from build123d import *

# Parameters (mm, degrees)
SKETCH_1_R          = 18.5
EXTRUDE_1_DEPTH     = 24
SKETCH_2_R          = 6
EXTRUDE_2_DEPTH     = 6
SKETCH_3_R          = 3
EXTRUDE_3_DEPTH     = 15.5
SKETCH_4_R          = 17.5
EXTRUDE_4_DEPTH     = 30
SKETCH_5_R          = 10
EXTRUDE_6_DEPTH     = 11.5
CUT_EXTRUDE_1_DEPTH = 12
SKETCH_7_R          = 1.5
CUT_EXTRUDE_2_DEPTH = 10


with BuildPart() as part:
    # 草图1 → 凸台-拉伸1 (new body)
    with BuildSketch(Plane(origin=(0, 0, 0), x_dir=(1, 0, 0), z_dir=(0, 1, 0))):
        with Locations(Location((0, 0, 0), (0, 0, 270))):
            Circle(SKETCH_1_R)
    extrude(amount=EXTRUDE_1_DEPTH)

    # 草图2 → 凸台-拉伸2 (add)
    with BuildSketch(Plane(origin=(0, 24, 0), x_dir=(1, 0, 0), z_dir=(0, 1, 0))):
        with Locations(Location((0, 7, 0), (0, 0, 270))):
            Circle(SKETCH_2_R)
    extrude(amount=EXTRUDE_2_DEPTH)

    # 草图3 → 凸台-拉伸3 (add)
    with BuildSketch(Plane(origin=(0, 30, 0), x_dir=(1, 0, 0), z_dir=(0, 1, 0))):
        with Locations(Location((0, 7, 0), (0, 0, 270))):
            Circle(SKETCH_3_R)
    extrude(amount=EXTRUDE_3_DEPTH)

    # 草图4 → 凸台-拉伸4 (add)
    with BuildSketch(Plane.XZ):
        with Locations(Location((0, 0, 0), (0, 0, 90))):
            Circle(SKETCH_4_R)
    extrude(amount=EXTRUDE_4_DEPTH)

    # 草图5 → 凸台-拉伸6 (add)
    with BuildSketch(Plane.XZ.offset(30)):
        with Locations(Location((0, 0, 0), (0, 0, 270))):
            Circle(SKETCH_5_R)
    extrude(amount=EXTRUDE_6_DEPTH)

    # 草图6 → 切除-拉伸1 (cut)
    with BuildSketch(Plane(origin=(0, 45.5, 0), x_dir=(1, 0, 0), z_dir=(0, 1, 0))):
        with BuildLine():
            Line((-3.711279789, 9.5), (4.099560016, 9.5))
            ThreePointArc((4.099560016, 9.5), (0.194140114, 13.405419903), (-3.711279789, 9.5))
        make_face()
    extrude(amount=-CUT_EXTRUDE_1_DEPTH, mode=Mode.SUBTRACT)

    # 草图7 → 切除-拉伸2 (cut)
    with BuildSketch(Plane(origin=(0, 24, 0), x_dir=(1, 0, 0), z_dir=(0, 1, 0))):
        with Locations(Location((-15.5, 0, 0), (0, 0, 270))):
            Circle(SKETCH_7_R)
        with Locations(Location((-7.75, 13.423393759, 0), (0, 0, 270))):
            Circle(SKETCH_7_R)
        with Locations(Location((7.75, 13.423393759, 0), (0, 0, 270))):
            Circle(SKETCH_7_R)
        with Locations(Location((15.5, 0, 0), (0, 0, 270))):
            Circle(SKETCH_7_R)
        with Locations(Location((7.75, -13.423393759, 0), (0, 0, 270))):
            Circle(SKETCH_7_R)
        with Locations(Location((-7.75, -13.423393759, 0), (0, 0, 270))):
            Circle(SKETCH_7_R)
    extrude(amount=-CUT_EXTRUDE_2_DEPTH, mode=Mode.SUBTRACT)


solid = part.part
Model file for the job. Use its own axes, mm. A direction names the side the tool comes from. Give positions to 0.01 mm unless a question says otherwise; leave off trailing zeros. Order: outer loops, then holes, each group sorted by start corner. A loop starts at its lowest first (then second) coordinate and runs counter-clockwise, first axis right, second up. Notation, with made-up numbers: M 43.5,21.25 L 59.5,21.25 A16 ccw 59.5,42.25 Z; hole C 1,75 d10. An arc over 180 degrees is marked long. Write item = value, one per line.
Q1. Flat gauge pins, fed straight in: pin 1 (6 mm diameter, centred on x = 12, z = 5.5, fed in from +Y); pin 2 (1.5 mm diameter, centred on x = 8, z = 13, fed in from +Y); pin 3 (1.7 mm diameter, centred on x = 0.5, y = 40.5, fed in from -Z). Where does each tip first touch, or does it go through?
Derived:
pin_1 = 24
pin_2 = 14
pin_3 = -9.5
Q2. Cut at D-D, the plane z = -5. List the corners of the cut face in (x, y).
Derived:
outline = M -17.81,0 L -16.77,0 L -16.77,-30 L -8.66,-30 L -8.66,-41.5 L 8.66,-41.5 L 8.66,-30 L 16.77,-30 L 16.77,0 L 17.81,0 L 17.81,24 L 5.66,24 L 5.66,30 L 2.24,30 L 2.24,45.5 L -2.24,45.5 L -2.24,30 L -5.66,30 L -5.66,24 L -17.81,24 Z
Q3. Cut at A-A, the plane x = 0. List the corners of the cut face in (y, z).
Derived:
outline = M -41.5,-10 L -30,-10 L -30,-17.5 L 0,-17.5 L 0,-18.5 L 24,-18.5 L 24,-13 L 30,-13 L 30,-10 L 33.5,-10 L 33.5,-9.5 L 45.5,-9.5 L 45.5,-4 L 30,-4 L 30,-1 L 24,-1 L 24,18.5 L 0,18.5 L 0,17.5 L -30,17.5 L -30,10 L -41.5,10 Z
Q4. Two-plate mould, pull along X, no slides. Class faces 4 (the cylindrical face through (-9.76, -35.67, 2.17)), 5 (the flat face through (0, 40, -9.5)), 6 (the cylindrical face through (-8.66, 19.07, 12.23)), 7 (the flat face through (16, 14, 0)): pulls with the +X half, pulls with the -X half, needs draft (parallel to the pull), parting line crosses it, or undercut.
Derived:
face_4 = parting line crosses it
face_5 = needs draft
face_6 = undercut
face_7 = undercut
Q5. Tool access for faces 1 (the flat face through (-8, 14, 13)), 2 (the flat face through (8, -30, 8)), 3 (the flat face through (0, -41.5, 0)): list every direction of +Z, -Z, +X, -X, +Y, -Y with a clear straight run to the whole face (end or side of a thin tool).
Derived:
face_1 = +Y
face_2 = -Y
face_3 = +Z, -Z, +X, -X, -Y
Q6. Cut at B-B, the plane z = 0. List the corners of the cut face in (x, y), then the cut area to 3 significant figures.
Derived:
outline = M -18.5,0 L -17.5,0 L -17.5,-30 L -10,-30 L -10,-41.5 L 10,-41.5 L 10,-30 L 17.5,-30 L 17.5,0 L 18.5,0 L 18.5,24 L 17,24 L 17,14 L 14,14 L 14,24 L -14,24 L -14,14 L -17,14 L -17,24 L -18.5,24 Z
area = 2,110 mm2
Q7. Cut at C-C, the plane y = 40. List the corners of the cut face in (x, z), then the cut area to 3 significant figures.
Derived:
outline = M -1.66,-9.5 L 1.66,-9.5 A3 ccw long Z
area = 27.1 mm2
Q8. Drill centre lines: line 1 (Z direction, x = 7, y = 18); line 2 (X direction, y = 14.5, z = 1); line 3 (Y direction, x = 1.5, z = 3). Where is each one in solid material? Low to high. Write a range as [from, to].
Derived:
line_1 = [-17.12, -14.72], [-12.12, 12.12], [14.72, 17.12]
line_2 = [-18.47, -16.62], [-14.38, 14.38], [16.62, 18.47]
line_3 = [-41.5, 24]
